Check sheet for the modelled part. Datum: model origin and axes. Units: mm. A direction names the side the tool comes from. Coordinates: 2 decimals unless noted, no trailing zeros. Write each loop counter-clockwise with the first axis right and the second up, starting at its lowest first coordinate (ties: lowest second). Pieces come first, ordered by that corner, then holes. Notation, with made-up numbers: M 57,50.25 L 66,50.25 A12 cw 66,70.25 Z; hole C -22,11 d3. An arc over 180 degrees is marked long. Answer as CSV lines item,"result". Start each with the question number.
Q1. Thickness scan on line 1 along X through (y, z) = (-6, 4.5) (3 decimals); line 2 along Y through (x, z) = (-30.5, 8.25); line 3 along Y through (x, z) = (0, 3.5). Record the ranges inside material, lowest first. Write a range as from..to.
Q2. Access from +Z, -Z, +X, -X, +Y, -Y to the whole of each face (thin tool, end or side, straight path). Record for faces 1 (the flat face through (-15.24, -33, 5)), 2 (the flat face through (0, -40.64, 5)), 3 (the flat face through (-50.8, -8, 5)), 4 (the flat face through (-31, 0, 5)).
Q3. Sectioned sample at A-A, the plane x = 0. Record the cut outline in (y, z) (3 decimals), then the cut area to 3 significant figures.
Q4. Sectioned sample at B-B, the plane y = -13. Record the cut outline in (x, z) (3 decimals).
Q5. Sectioned sample at C-C, the plane z = 7. Record the cut outline in (x, y) (1 decimal).
Q6. Sectioned sample at D-D, the plane x = -45. Record the cut outline in (y, z) (3 decimals), then the cut area to 3 significant figures.
Q7. Depth check by flat-ended pin: pin 1 Ø2.5 at (y, z) = (-32.5, 5.5) entering from -X; pin 2 Ø5 at (x, z) = (-17, 7.5) entering from +Y; pin 3 Ø4 at (x, z) = (-16.5, 2.5) entering from -Y; pin 4 Ø0.8 at (x, y) = (-28.65, -24.97) entering from +Z. Enter the tip coordinate at first touch or a pass-through.
Q8. Mould release check, pull along Y, two halves, no side actions. Record for faces 5 (the cylindrical face through (-0.86, -3.874, 4.696)), 6 (the flat face through (-46, -15.24, 5)), 7 (the flat face through (-15, -8, 0)), 8 (the cylindrical face through (-13.712, -39.191, 4.829)): pulls with the +Y half, pulls with the -Y half, needs draft (parallel to the pull), parting line crosses it, or undercut.
from build123d import *

# Parameters (mm, degrees)
SKETCH1_R           = 3.96875
BOSS_EXTRUDE1_DEPTH = 9.525
FILLET2_R           = 5.08
CUT_EXTRUDE1_REACH  = 11.525
SKETCH2_R           = 0.635


with BuildPart() as part:
    # Sketch1 → Boss-Extrude1 (new body)
    with BuildSketch(Plane.XY):
        Polygon((-15.24, -40.64), (15.24, -40.64), (15.24, 40.64), (-15.24, 40.64), (-15.24, 0), (-41.275, 0), (-41.275, -15.24), (-50.8, -15.24), (-50.8, 0), (-60.325, 0), (-60.325, -30.48), (-15.24, -30.48), align=None)
        Circle(SKETCH1_R, mode=Mode.SUBTRACT)
    extrude(amount=BOSS_EXTRUDE1_DEPTH)

    # Fillet2
    fillet2_edges = [part.edges().sort_by_distance(p)[0] for p in [
        (-15.24, 0, 4.7625),
        (-15.24, 40.64, 4.7625),
        (15.24, 40.64, 4.7625),
        (15.24, -40.64, 4.7625),
        (-15.24, -40.64, 4.7625),
    ]]
    fillet(fillet2_edges, radius=FILLET2_R)

    # Sketch2 → Cut-Extrude1 (cut, up to next)
    with BuildSketch(Plane.XY.offset(9.525), mode=Mode.PRIVATE) as cut_extrude1_sk1:
        with Locations((-28.6512, -8.683)):
            Circle(SKETCH2_R)
    cut_extrude1_tool1 = extrude(cut_extrude1_sk1.sketch, amount=-CUT_EXTRUDE1_REACH, mode=Mode.PRIVATE) & part.part
    add(cut_extrude1_tool1.solids().sort_by_distance((-28.6512, -8.683, 9.525))[0], mode=Mode.SUBTRACT)
    # Sketch2 → Cut-Extrude1 (cut, up to next)
    with BuildSketch(Plane.XY.offset(9.525), mode=Mode.PRIVATE) as cut_extrude1_sk2:
        with Locations((-28.6512, -16.825545611)):
            Circle(SKETCH2_R)
    cut_extrude1_tool2 = extrude(cut_extrude1_sk2.sketch, amount=-CUT_EXTRUDE1_REACH, mode=Mode.PRIVATE) & part.part
    add(cut_extrude1_tool2.solids().sort_by_distance((-28.6512, -16.825546, 9.525))[0], mode=Mode.SUBTRACT)
    # Sketch2 → Cut-Extrude1 (cut, up to next)
    with BuildSketch(Plane.XY.offset(9.525), mode=Mode.PRIVATE) as cut_extrude1_sk3:
        with Locations((-28.6512, -24.968091222)):
            Circle(SKETCH2_R)
    cut_extrude1_tool3 = extrude(cut_extrude1_sk3.sketch, amount=-CUT_EXTRUDE1_REACH, mode=Mode.PRIVATE) & part.part
    add(cut_extrude1_tool3.solids().sort_by_distance((-28.6512, -24.968091, 9.525))[0], mode=Mode.SUBTRACT)


solid = part.part
Output:
1,line 1,"x = -60.325..-50.8, -41.275..15.24"
1,line 2,"y = -30.48..0"
1,line 3,"y = -40.64..-3.97, 3.97..40.64"
2,face 1,"+Z, -Z, -X, -Y"
2,face 2,"+Z, -Z, +X, -X, -Y"
2,face 3,"+Z, -Z, +Y"
2,face 4,"+Z, -Z, -X, +Y"
3,outline,"M -40.64,0 L -3.969,0 L -3.969,9.525 L -40.64,9.525 Z; M 3.969,0 L 40.64,0 L 40.64,9.525 L 3.969,9.525 Z"
3,area,"699 mm^2"
4,outline,"M -60.325,0 L -50.8,0 L -50.8,9.525 L -60.325,9.525 Z; M -41.275,0 L 15.24,0 L 15.24,9.525 L -41.275,9.525 Z"
5,outline,"M -60.3,-30.5 L -15.2,-30.5 L -15.2,-35.6 A5.1 ccw -10.2,-40.6 L 10.2,-40.6 A5.1 ccw 15.2,-35.6 L 15.2,35.6 A5.1 ccw 10.2,40.6 L -10.2,40.6 A5.1 ccw -15.2,35.6 L -15.2,5.1 A5.1 cw -20.3,0 L -41.3,0 L -41.3,-15.2 L -50.8,-15.2 L -50.8,0 L -60.3,0 Z; hole C -28.7,-25 d1.3; hole C -28.7,-16.8 d1.3; hole C -28.7,-8.7 d1.3; hole C 0,0 d7.9"
6,outline,"M -30.48,0 L -15.24,0 L -15.24,9.525 L -30.48,9.525 Z"
6,area,"145 mm^2"
7,pin 1,"stops at x = -15.24"
7,pin 2,"stops at y = 38.2"
7,pin 3,"stops at y = -38.2"
7,pin 4,"passes through"
8,face 5,"undercut"
8,face 6,"pulls with the +Y half"
8,face 7,"needs draft"
8,face 8,"pulls with the -Y half"
